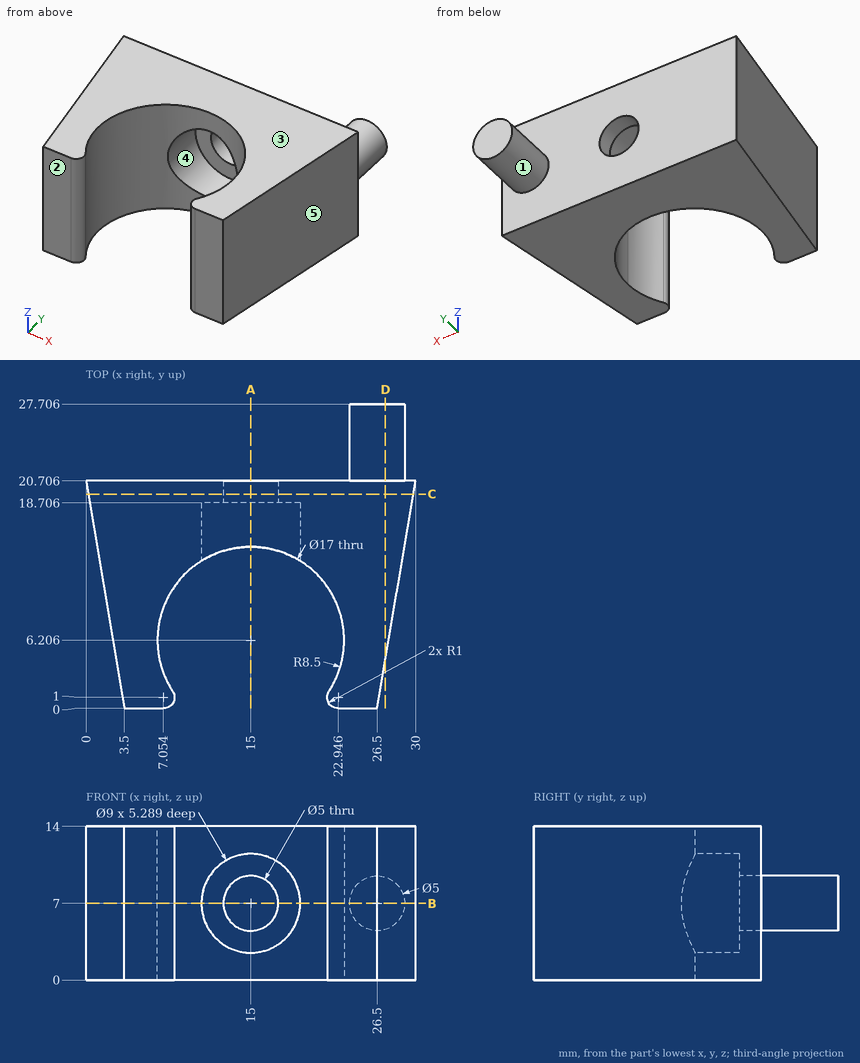
Can you work these out from the drawing? Everything is in mm from the part's minimum corner. A direction names the side the tool comes from. Coordinates: 2 decimals unless noted, no trailing zeros. Write each loop counter-clockwise with the first axis right and the second up, starting at its lowest first coordinate (ties: lowest second). Pieces come first, ordered by that corner, then holes. Notation, with made-up numbers: (-4, 42) -> (27, 42) arc R20 ccw to (27, 81) -> close; hole circle Ø10 at (21, 10.25). An arc over 180 degrees is marked (long way). Write item = value, one per line.
(1) Thinking about a two-plate mould opening in X: for the marked faces 3, 4 and 5, which applies, +X half, -X half, draft (parallel to the pull), parting line (faces both ways), or undercut?
Verdict:
face_3 = draft
face_4 = undercut
face_5 = +X half
(2) On a 3-axis mill with a long thin cutter (end or side, diameter ignored), from which of +Z, -Z, +X, -X, +Y, -Y can I reach the whole of each face in a straight line? I mean the marked faces 1 and 2. Say none if no direction works.
Verdict:
face_1 = +Y
face_2 = +Z, -Z, +X, -X, -Y
(3) Imagine slicing it at D-D (x = 27.25). Please give me the cut outline in (y, z) (1 decimal).
Verdict:
outline = (4.4, 0) -> (20.7, 0) -> (20.7, 4.6) -> (27.7, 4.6) -> (27.7, 9.4) -> (20.7, 9.4) -> (20.7, 14) -> (4.4, 14) -> close
(4) If I drill on probe 1 along Z at (x, y) = (15, 20.05); probe 2 along Y at (x, z) = (3.75, 2.25); probe 3 along Z at (x, y) = (15, 15.25), over which ranges is the centre line in solid material (lowest first)?
Verdict:
probe_1 = 0 to 4.5, 9.5 to 14
probe_2 = 0 to 20.71
probe_3 = 0 to 2.5, 11.5 to 14
(5) Imagine slicing it at C-C (y = 19.5). Please give me the cut outline in (x, z).
Verdict:
outline = (0.2, 0) -> (29.8, 0) -> (29.8, 14) -> (0.2, 14) -> close; hole circle Ø5 at (15, 7)
(6) For pin 1 (4 mm diameter, centred on x = 10, z = 5.5, fed in from +Y); pin 2 (6 mm diameter, centred on x = 18.5, z = 7, fed in from -Y) (1 decimal); pin 3 (8 mm diameter, centred on x = 15, y = 7.5, fed in from -Z); pin 4 (1 mm diameter, centred on y = 18.5, z = 5.5, fed in from -X), each with a flat end and sliding along its axis, tell me the tip position at first contact or that it passes through.
Verdict:
pin_1 = 20.71
pin_2 = 11.7
pin_3 = through
pin_4 = 0.29
(7) Imagine slicing it at B-B (z = 7). Please give me the cut outline in (x, y).
Verdict:
outline = (0, 20.71) -> (3.5, 0) -> (7.05, 0) arc R1 ccw to (7.89, 1.55) arc R8.5 cw to (10.5, 13.42) -> (10.5, 18.71) -> (12.5, 18.71) -> (12.5, 20.71) -> close; (17.5, 18.71) -> (19.5, 18.71) -> (19.5, 13.42) arc R8.5 cw to (22.11, 1.55) arc R1 ccw to (22.95, 0) -> (26.5, 0) -> (30, 20.71) -> (29, 20.71) -> (29, 27.71) -> (24, 27.71) -> (24, 20.71) -> (17.5, 20.71) -> close
(8) Imagine slicing it at A-A (x = 15). Please give me the cut outline in (y, z).
Verdict:
outline = (14.71, 0) -> (20.71, 0) -> (20.71, 4.5) -> (18.71, 4.5) -> (18.71, 2.5) -> (14.71, 2.5) -> close; (14.71, 11.5) -> (18.71, 11.5) -> (18.71, 9.5) -> (20.71, 9.5) -> (20.71, 14) -> (14.71, 14) -> close
